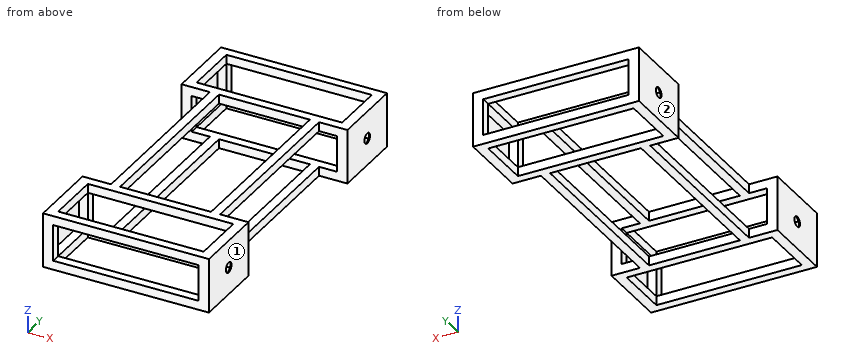
from build123d import *

# Parameters (mm, degrees)
F0_W      = 406.4
F0_H      = 152.4
F0_W_2    = 25.4
F0_H_2    = 508
F1_DEPTH  = 25.4
F2_W      = 25.4
F2_H      = 25.4
F3_DEPTH  = 101.6
F4_W      = 25.4
F4_H      = 508
F5_DEPTH  = 25.4
F6_W      = 203.2
F6_H      = 152.4
F7_DEPTH  = 3.175
F8_W      = 203.2
F8_H      = 152.4
F9_DEPTH  = 3.175
F10_R     = 14.2875
F11_DEPTH = 463.551


with BuildPart() as f1:
    # F0 (on Top) → F1 (new body)
    with BuildSketch(Plane.XY):
        Polygon((228.6, 457.2), (-228.6, 457.2), (-228.6, 254), (-203.2, 254), (-152.4, 254), (-127, 254), (127, 254), (152.4, 254), (203.2, 254), (228.6, 254), align=None)
        with Locations((0, 355.6)):
            Rectangle(F0_W, F0_H, mode=Mode.SUBTRACT)
        with Locations((-139.7, 0)):
            Rectangle(F0_W_2, F0_H_2)
        with Locations((139.7, 0)):
            Rectangle(F0_W_2, F0_H_2)
        Polygon((-127, -254), (-152.4, -254), (-203.2, -254), (-203.2, -279.4), (203.2, -279.4), (203.2, -254), (152.4, -254), (127, -254), align=None)
        Polygon((-203.2, -279.4), (-203.2, -254), (-228.6, -254), (-228.6, -457.2), (228.6, -457.2), (228.6, -254), (203.2, -254), (203.2, -279.4), (203.2, -431.8), (-203.2, -431.8), align=None)
    extrude(amount=F1_DEPTH)

    # F2 (on face) → F3 (join)
    with BuildSketch(Plane.XY.offset(25.4)):
        with Locations((-215.9, -444.5)):
            Rectangle(F2_W, F2_H)
        with Locations((-215.9, 444.5)):
            Rectangle(F2_W, F2_H)
        with Locations((215.9, 444.5)):
            Rectangle(F2_W, F2_H)
        with Locations((215.9, -444.5)):
            Rectangle(F2_W, F2_H)
        with Locations((-215.9, -266.7)):
            Rectangle(F2_W, F2_H)
        with Locations((-215.9, 266.7)):
            Rectangle(F2_W, F2_H)
        with Locations((215.9, -266.7)):
            Rectangle(F2_W, F2_H)
        with Locations((215.9, 266.7)):
            Rectangle(F2_W, F2_H)
    extrude(amount=F3_DEPTH)

    # F4 (on face) → F5 (join)
    with BuildSketch(Plane.XY.offset(127)):
        Polygon((228.6, 431.8), (228.6, 457.2), (-228.6, 457.2), (-228.6, 431.8), (-203.2, 431.8), (203.2, 431.8), align=None)
        Polygon((228.6, 254), (228.6, 431.8), (203.2, 431.8), (203.2, 279.4), (203.2, 254), align=None)
        Polygon((-203.2, 431.8), (-228.6, 431.8), (-228.6, 254), (-203.2, 254), (-203.2, 279.4), align=None)
        Polygon((203.2, 254), (203.2, 279.4), (-203.2, 279.4), (-203.2, 254), (-152.4, 254), (-127, 254), (127, 254), (152.4, 254), align=None)
        with Locations((139.7, 0)):
            Rectangle(F4_W, F4_H)
        with Locations((-139.7, 0)):
            Rectangle(F4_W, F4_H)
        Polygon((203.2, -254), (152.4, -254), (127, -254), (-127, -254), (-152.4, -254), (-203.2, -254), (-203.2, -279.4), (203.2, -279.4), align=None)
        Polygon((228.6, -254), (203.2, -254), (203.2, -279.4), (203.2, -431.8), (228.6, -431.8), align=None)
        Polygon((-203.2, -279.4), (-203.2, -254), (-228.6, -254), (-228.6, -431.8), (-203.2, -431.8), align=None)
        Polygon((228.6, -457.2), (228.6, -431.8), (203.2, -431.8), (-203.2, -431.8), (-228.6, -431.8), (-228.6, -457.2), align=None)
    extrude(amount=F5_DEPTH)

    # F6 (on face) → F7 (join)
    with BuildSketch(Plane.YZ.offset(228.6)):
        with Locations((-355.6, 76.2)):
            Rectangle(F6_W, F6_H)
        with Locations((355.6, 76.2)):
            Rectangle(F6_W, F6_H)
    extrude(amount=F7_DEPTH)

    # F8 (on face) → F9 (join)
    with BuildSketch(Plane(origin=(-228.6, 0, 0), x_dir=(0, -1, 0), z_dir=(-1, 0, 0))):
        with Locations((-355.6, 76.2)):
            Rectangle(F8_W, F8_H)
        with Locations((355.6, 76.2)):
            Rectangle(F8_W, F8_H)
    extrude(amount=F9_DEPTH)

    # F10 (on face) → F11 (cut, through all)
    with BuildSketch(Plane.YZ.offset(231.775)):
        with Locations((355.6, 76.2)):
            Circle(F10_R)
        with Locations((-355.6, 76.2)):
            Circle(F10_R)
    extrude(amount=-F11_DEPTH, mode=Mode.SUBTRACT)


solid = f1.part
Could you check a few things on this model? Use its own coordinates, in mm. Face numbers are marked on the shaded views. Give positions to 0.01 mm unless a question says otherwise; leave off trailing zeros. Write each loop counter-clockwise with the first axis right and the second up, starting at its lowest first coordinate (ties: lowest second). Pieces come first, ordered by that corner, then holes. Notation, with made-up numbers: (2, 42.25) - (30, 42.25) arc R31 cw to (30, 77.25) - close; hole circle Ø6 at (-13, 73.5). An arc over 180 degrees is marked (long way). Use CSV: the item, a comma, the result in double quotes. Start each with the question number.
Item 1: I'm going to push flat-ended pins straight in: pin 1 (7.5 mm diameter, centred on x = -215.5, y = -385.5, fed in from -Z); pin 2 (12.5 mm diameter, centred on y = 92, z = 13.5, fed in from +X); pin 3 (20.5 mm diameter, centred on y = 102.5, z = 142, fed in from -X); pin 4 (12 mm diameter, centred on y = -39, z = 37, fed in from +X). Where does each tip first touch, or does it pass through?
Item 2: I want a section at D-D, the plane y = -299.5. Please give me the cut outline in (x, z) (3 decimals).
Item 3: If I drill on line 1 along Y through (x, z) = (210, 98); line 2 along X through (y, z) = (372, 72) (3 decimals); line 3 along X through (y, z) = (-387.5, 144) (3 decimals), over which ranges is the centre line in solid material (lowest first)?
Item 4: If we mould it in two halves opening along X, with no side actions, what happens to the marked faces 1 and 2? For each: pulls with the +X half, pulls with the -X half, needs draft (parallel to the pull), parting line crosses it, or undercut.
Item 5: I want a section at C-C, the plane z = 137.5. Please give me the cut outline in (x, y) (3 decimals).
Item 6: I want a section at A-A, the plane x = -102. Give the number of separate pieces and of enclosed holes in the cut face, then the cut area to 3 significant figures.
Item 7: I want a section at B-B, the plane y = 11. Please give me the cut outline in (x, z).
Findings:
1,pin 1,"stops at z = 0"
1,pin 2,"stops at x = 152.4"
1,pin 3,"stops at x = -152.4"
1,pin 4,"passes through"
2,outline,"(-231.775, 0) - (-203.2, 0) - (-203.2, 25.4) - (-228.6, 25.4) - (-228.6, 127) - (-203.2, 127) - (-203.2, 152.4) - (-231.775, 152.4) - close; (203.2, 0) - (231.775, 0) - (231.775, 152.4) - (203.2, 152.4) - (203.2, 127) - (228.6, 127) - (228.6, 25.4) - (203.2, 25.4) - close"
3,line 1,"y = -457.2 to -431.8, -279.4 to -254, 254 to 279.4, 431.8 to 457.2"
3,line 2,"x = -231.775 to -228.6, 228.6 to 231.775"
3,line 3,"x = -231.775 to -203.2, 203.2 to 231.775"
4,face 1,"pulls with the +X half"
4,face 2,"pulls with the -X half"
5,outline,"(-231.775, -457.2) - (231.775, -457.2) - (231.775, -254) - (152.4, -254) - (152.4, 254) - (231.775, 254) - (231.775, 457.2) - (-231.775, 457.2) - (-231.775, 254) - (-152.4, 254) - (-152.4, -254) - (-231.775, -254) - close; hole (-203.2, -431.8) - (203.2, -431.8) - (203.2, -279.4) - (-203.2, -279.4) - close; hole (-203.2, 279.4) - (203.2, 279.4) - (203.2, 431.8) - (-203.2, 431.8) - close; hole (-127, -254) - (127, -254) - (127, 254) - (-127, 254) - close"
6,separate pieces,"8"
6,enclosed holes,"0"
6,area,"5,160 mm2"
7,outline,"(-152.4, 0) - (-127, 0) - (-127, 25.4) - (-152.4, 25.4) - close; (-152.4, 127) - (-127, 127) - (-127, 152.4) - (-152.4, 152.4) - close; (127, 0) - (152.4, 0) - (152.4, 25.4) - (127, 25.4) - close; (127, 127) - (152.4, 127) - (152.4, 152.4) - (127, 152.4) - close"
